from build123d import *

# Parameters (mm, degrees)
BOSS_EXTRUDE2_DEPTH = 152.4
SHELL1_T            = -1.5875
SKETCH4_W           = 25.4
SKETCH4_H           = 12.7
CUT_EXTRUDE1_DEPTH  = 152.4


with BuildPart() as part:
    # Sketch3 → Boss-Extrude2 (new body)
    with BuildSketch(Plane.XY):
        Polygon((-228.6, 127), (0, 50.8), (0, 0), (-228.6, 0), align=None)
    extrude(amount=BOSS_EXTRUDE2_DEPTH)

    # Shell1
    shell1_openings = [part.faces().sort_by_distance(p)[0] for p in [
        (-114.3, 0, 76.2),
    ]]
    offset(amount=SHELL1_T, openings=shell1_openings, kind=Kind.INTERSECTION)

    # Sketch4 → Cut-Extrude1 (cut)
    with BuildSketch(Plane(origin=(0, 0, 0), x_dir=(-1, 0, 0), z_dir=(0, 0, -1))):
        with Locations((215.9, 6.35)):
            Rectangle(SKETCH4_W, SKETCH4_H)
    extrude(amount=-CUT_EXTRUDE1_DEPTH, mode=Mode.SUBTRACT)


solid = part.part
For this review, take the finished solid that the model builds, in its own axes (mm). A direction names the side the tool comes from. Coordinates: 2 decimals unless noted, no trailing zeros. Loops run counter-clockwise (first coordinate to the right, second up) from the corner with the lowest first, then second, coordinate; pieces in that order, holes last. Notation, with made-up numbers: (-27.75, 0) -> (-3.75, 0) arc R13 cw to (-3.75, 11) -> close; hole circle Ø11 at (87, 47). An arc over 180 degrees is marked (long way). Write each question's results on one line, items separated by ' | '.
Q1. For pin 1 Ø0.5 at (y, z) = (5, 152) entering from -X; pin 2 Ø1 at (x, z) = (-24, 54) entering from +Y; pin 3 Ø4 at (x, z) = (-167.5, 101) entering from +Y; pin 4 Ø6 at (x, y) = (-145, 81) entering from -Z, all flat-tipped, find the tip position at first contact; note any pin that passes through.
Taken from the geometry:
pin 1: x = -203.2 | pin 2: y = 58.97 | pin 3: y = 107.3 | pin 4: z = 0
Q2. To check wall thickness, follow line 1 along Z through (x, y) = (-15.5, 50); line 2 along X through (y, z) = (43, 41); line 3 along X through (y, z) = (10.5, 107.5). State the ranges of each line that lie inside material, in increasing order. Write a range as [from, to].
Taken from the geometry:
line 1: [0, 1.59], [150.81, 152.4] | line 2: [-228.6, -227.01], [-1.59, 0] | line 3: [-1.59, 0]
Q3. Add section C-C, the plane x = -91.5. State the section outline as (y, z) points.
Taken from the geometry:
outline: (0, 0) -> (81.3, 0) -> (81.3, 152.4) -> (0, 152.4) -> (0, 150.81) -> (79.63, 150.81) -> (79.63, 1.59) -> (0, 1.59) -> close
Q4. Mouldability with a two-part tool opening along Z and no side actions: class faces 1 (the flat face through (-115.878, 87.753, 75.155)), 2 (the flat face through (-138, 50, 152.4)), 3 (the flat face through (-138, 50, 0)), 4 (the flat face through (-1.588, 25, 75)) as +Z half, -Z half, draft (parallel to the pull), parting line (faces both ways), or undercut.
Taken from the geometry:
face 1: undercut | face 2: +Z half | face 3: -Z half | face 4: undercut
Q5. Add section D-D, the plane y = 97.5. State the section outline as (x, z) points.
Taken from the geometry:
outline: (-228.6, 0) -> (-140.1, 0) -> (-140.1, 152.4) -> (-228.6, 152.4) -> close; hole (-227.01, 1.59) -> (-145.12, 1.59) -> (-145.12, 150.81) -> (-227.01, 150.81) -> close
Q6. Add section A-A, the plane y = 30.5. State the section outline as (x, z) points.
Taken from the geometry:
outline: (-228.6, 0) -> (0, 0) -> (0, 152.4) -> (-228.6, 152.4) -> close; hole (-227.01, 1.59) -> (-1.59, 1.59) -> (-1.59, 150.81) -> (-227.01, 150.81) -> close
Q7. Add section B-B, the plane z = 22.5. State the section outline as (x, y) points.
Taken from the geometry:
outline: (-228.6, 12.7) -> (-227.01, 12.7) -> (-227.01, 124.8) -> (-1.59, 49.66) -> (-1.59, 0) -> (0, 0) -> (0, 50.8) -> (-228.6, 127) -> close
Q8. Machinability: for faces 5 (the flat face through (0, 26, 75)), 6 (the flat face through (-227.012, 68, 75)), 7 (the flat face through (-228, 12.7, 76)), which of the approach directions +Z, -Z, +X, -X, +Y, -Y give a long, thin tool a straight path to every point of the face, cutting with its end or side? Answer none if there is none.
Taken from the geometry:
face 5: +Z, -Z, +X, +Y, -Y | face 6: -Y | face 7: +Z, -Z, -X, -Y
